Can you work these out from the model? Positions are in its coordinate system, mm. A direction names the side the tool comes from. Round coordinates to 2 decimals unless told otherwise and drop trailing zeros. Order: outer loops, then holes, each group sorted by start corner. A loop starts at its lowest first (then second) coordinate and runs counter-clockwise, first axis right, second up. Notation, with made-up numbers: M 29,66.5 L 58,66.5 A18 cw 58,73.5 Z; hole C 6.25,70.5 d7. An arc over 180 degrees is marked long. One line per question, with ' | ' between items.
```python
from build123d import *

# Parameters (mm, degrees)
SKETCH1_W                       = 90
SKETCH1_H                       = 54
BOSS_EXTRUDE1_DEPTH             = 38
CUT_EXTRUDE1_START              = -15.5
CUT_EXTRUDE1_DEPTH              = 13
SKETCH4_W                       = 13
SKETCH4_H                       = 4.8
CUT_EXTRUDE2_DEPTH              = 14
SKETCH3_R                       = 19.5
CUT_EXTRUDE3_DEPTH              = 8
SKETCH7_R                       = 1.5
CUT_EXTRUDE4_DEPTH              = 5
M5X0_8_TAPPED_HOLE1_D           = 4.2
M5X0_8_TAPPED_HOLE1_DEPTH       = 8
M5X0_8_TAPPED_HOLE1_CSINK_D     = 6
M5X0_8_TAPPED_HOLE1_CSINK_ANGLE = 90
M5X0_8_TAPPED_HOLE1_TIP         = 1.2618073


with BuildPart() as part:
    # Sketch1 → Boss-Extrude1 (new body)
    with BuildSketch(Plane(origin=(0, 0, 0), x_dir=(1, 0, 0), z_dir=(0, 1, 0))):
        Rectangle(SKETCH1_W, SKETCH1_H)
    extrude(amount=BOSS_EXTRUDE1_DEPTH)

    # Sketch2 → Cut-Extrude1 (cut)
    with BuildSketch(Plane.ZY.offset(45).offset(CUT_EXTRUDE1_START)):
        Polygon((-4.9, 2.5), (18.6, 2.5), (18.6, 21.5), (23.4, 21.5), (23.4, 24), (18.6, 24), (18.6, 37.402398481), (-4.9, 37.402398481), (-4.9, 24), (-9.7, 24), (-9.7, 21.5), (-4.9, 21.5), align=None)
    cut_extrude1 = extrude(amount=-CUT_EXTRUDE1_DEPTH, mode=Mode.SUBTRACT)

    # Sketch4 → Cut-Extrude2 (cut)
    with BuildSketch(Plane.XZ.offset(-24)):
        with Locations((-23, 21)):
            Rectangle(SKETCH4_W, SKETCH4_H)
        with Locations((-23, -7.3)):
            Rectangle(SKETCH4_W, SKETCH4_H)
    cut_extrude2 = extrude(amount=-CUT_EXTRUDE2_DEPTH, mode=Mode.SUBTRACT)

    # Sketch3 → Cut-Extrude3 (cut)
    with BuildSketch(Plane(origin=(0, 38, 0), x_dir=(1, 0, 0), z_dir=(0, 1, 0))):
        with Locations((-23, -1)):
            Circle(SKETCH3_R)
    cut_extrude3 = extrude(amount=-CUT_EXTRUDE3_DEPTH, mode=Mode.SUBTRACT)

    # Sketch7 → Cut-Extrude4 (cut)
    with BuildSketch(Plane(origin=(0, 21.5, 0), x_dir=(1, 0, 0), z_dir=(0, 1, 0))):
        with Locations((-23, 7.507766872)):
            Circle(SKETCH7_R)
        with Locations((-23, -19.255354552)):
            Circle(SKETCH7_R)
    cut_extrude4 = extrude(amount=-CUT_EXTRUDE4_DEPTH, mode=Mode.SUBTRACT)

    # Mirror1: Cut-Extrude1, Cut-Extrude2, Cut-Extrude3, Cut-Extrude4 across plane
    add(cut_extrude1.mirror(Plane(origin=(0, 0, 0), x_dir=(0, 0, 1), z_dir=(1, 0, 0))), mode=Mode.SUBTRACT)
    add(cut_extrude2.mirror(Plane(origin=(0, 0, 0), x_dir=(0, 0, 1), z_dir=(1, 0, 0))), mode=Mode.SUBTRACT)
    add(cut_extrude3.mirror(Plane(origin=(0, 0, 0), x_dir=(0, 0, 1), z_dir=(1, 0, 0))), mode=Mode.SUBTRACT)
    add(cut_extrude4.mirror(Plane(origin=(0, 0, 0), x_dir=(0, 0, 1), z_dir=(1, 0, 0))), mode=Mode.SUBTRACT)

    # M5x0.8 Tapped Hole1
    with Locations(Plane(origin=(23, 34, -27), x_dir=(-1, 0, 0), z_dir=(0, 0, -1))):
        with Locations((0, 0), (46, 0)):
            CounterSinkHole(M5X0_8_TAPPED_HOLE1_D / 2, M5X0_8_TAPPED_HOLE1_CSINK_D / 2, depth=M5X0_8_TAPPED_HOLE1_DEPTH, counter_sink_angle=M5X0_8_TAPPED_HOLE1_CSINK_ANGLE)
            with Locations((0, 0, -(M5X0_8_TAPPED_HOLE1_DEPTH + M5X0_8_TAPPED_HOLE1_TIP / 2))):  # 118° drill point
                Cone(0, M5X0_8_TAPPED_HOLE1_D / 2, M5X0_8_TAPPED_HOLE1_TIP, mode=Mode.SUBTRACT)


solid = part.part
```
(1) Please list where these lines run through material, in increasing order: probe 1 along X at (y, z) = (22, -6.5); probe 2 along Z at (x, y) = (-23, 17.8); probe 3 along Z at (x, y) = (22.5, 15). Write a range as [from, to].
Final values:
probe 1: [-45, -29.5], [-16.5, 16.5], [29.5, 45] | probe 2: [-27, -9.01], [-6.01, -4.9], [20.76, 27] | probe 3: [-27, -4.9], [18.6, 27]
(2) If we section it at A-A on y = 12.5: Please give me the cut outline in (x, z), plus the area to 3 significant figures.
Final values:
outline: M -45,-27 L 45,-27 L 45,27 L -45,27 Z; hole M -29.5,-4.9 L -16.5,-4.9 L -16.5,18.6 L -29.5,18.6 Z; hole M 16.5,-4.9 L 29.5,-4.9 L 29.5,18.6 L 16.5,18.6 Z | area: 4,250 mm^2
(3) Will these pins go through, and if not, where does the flat tip stop? pin 1 Ø2.5 at (x, z) = (-22.5, 19.5) entering from +Y; pin 2 Ø14.5 at (x, y) = (23, 32) entering from -Z; pin 3 Ø2 at (x, z) = (30.5, 13) entering from +Y; pin 4 Ø0.9 at (x, z) = (-22.5, -8) entering from +Y.
Final values:
pin 1: y = 21.5 | pin 2: z = -27 | pin 3: y = 30 | pin 4: y = 16.5
(4) If we section it at D-D on x = -23: Please give me the cut outline in (y, z), plus the area to 3 significant figures.
Final values:
outline: M 0,-27 L 31,-27 L 31.9,-26.1 L 31.9,-19 L 32.73,-18.5 L 30,-18.5 L 30,-9.7 L 21.5,-9.7 L 21.5,-9.01 L 16.5,-9.01 L 16.5,-6.01 L 21.5,-6.01 L 21.5,-4.9 L 2.5,-4.9 L 2.5,18.6 L 16.5,18.6 L 16.5,20.76 L 21.5,20.76 L 21.5,23.4 L 38,23.4 L 38,27 L 0,27 Z; M 35.27,-18.5 L 36.1,-19 L 36.1,-26.1 L 37,-27 L 38,-27 L 38,-18.5 Z | area: 927 mm^2
(5) If we section it at B-B on x = 30.5: Please give me the cut outline in (y, z), plus the area to 3 significant figures.
Final values:
outline: M 0,-27 L 38,-27 L 38,-17 L 30,-17 L 30,19 L 38,19 L 38,27 L 0,27 Z | area: 1,760 mm^2
(6) If we section it at C-C on z = 12.5: Please give me the cut outline in (x, y), plus the area to 3 significant figures.
Final values:
outline: M -45,0 L 45,0 L 45,38 L 38.75,38 L 38.75,30 L 29.5,30 L 29.5,2.5 L 16.5,2.5 L 16.5,30 L 7.25,30 L 7.25,38 L -7.25,38 L -7.25,30 L -16.5,30 L -16.5,2.5 L -29.5,2.5 L -29.5,30 L -38.75,30 L -38.75,38 L -45,38 Z | area: 2,200 mm^2
(7) On a 3-axis mill with a long thin cutter (end or side, diameter ignored), from which of +Z, -Z, +X, -X, +Y, -Y can I reach the whole of each face in a straight line? I mean faces 1 (the cylindrical face through (-23.325, 19.035, -6.043)), 2 (the flat face through (-1, 38, 0)). Say none if no direction works.
Final values:
face 1: +Y | face 2: +Z, -Z, +X, -X, +Y
